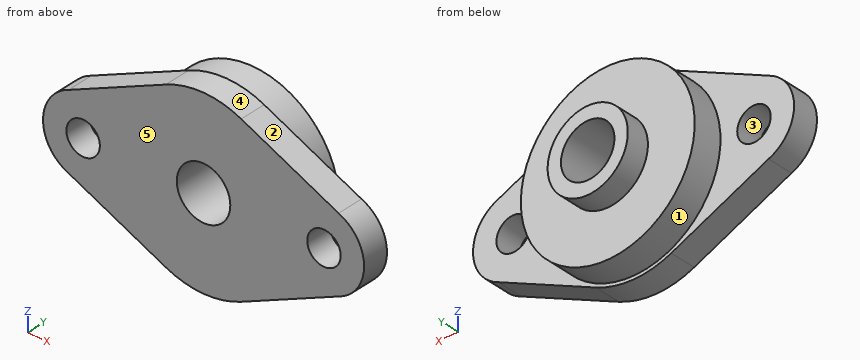
from build123d import *

# Parameters (mm, degrees)
SKETCH1_R           = 2.5
SKETCH1_R_2         = 4
BOSS_EXTRUDE1_DEPTH = 4
SKETCH2_R           = 13
SKETCH2_R_2         = 4
BOSS_EXTRUDE2_DEPTH = 4.5
SKETCH3_R           = 6
SKETCH3_R_2         = 4
BOSS_EXTRUDE3_DEPTH = 3.5


with BuildPart() as part:
    # Sketch1 → Boss-Extrude1 (new body)
    with BuildSketch(Plane(origin=(0, 0, 0), x_dir=(1, 0, 0), z_dir=(0, 1, 0))):
        with BuildLine():
            Line((-20.189639751, 5.586186334), (-5.632256707, 12.268972426))
            ThreePointArc((-5.632256707, 12.268972426), (0, 13.5), (5.632256707, 12.268972426))
            Line((5.632256707, 12.268972426), (20.189639751, 5.586186334))
            ThreePointArc((20.189639751, 5.586186334), (24, 0), (20.189639751, -5.586186334))
            Line((20.189639751, -5.586186334), (5.632256707, -12.268972426))
            ThreePointArc((5.632256707, -12.268972426), (0, -13.5), (-5.632256707, -12.268972426))
            Line((-5.632256707, -12.268972426), (-20.189639751, -5.586186334))
            ThreePointArc((-20.189639751, -5.586186334), (-24, 0), (-20.189639751, 5.586186334))
        make_face()
        with Locations((18, 0)):
            Circle(SKETCH1_R, mode=Mode.SUBTRACT)
        with Locations((-18, 0)):
            Circle(SKETCH1_R, mode=Mode.SUBTRACT)
        Circle(SKETCH1_R_2, mode=Mode.SUBTRACT)
    extrude(amount=BOSS_EXTRUDE1_DEPTH)

    # Sketch2 → Boss-Extrude2 (add)
    with BuildSketch(Plane(origin=(0, 4, 0), x_dir=(1, 0, 0), z_dir=(0, 1, 0))):
        Circle(SKETCH2_R)
        Circle(SKETCH2_R_2, mode=Mode.SUBTRACT)
    extrude(amount=BOSS_EXTRUDE2_DEPTH)

    # Sketch3 → Boss-Extrude3 (add)
    with BuildSketch(Plane(origin=(0, 8.5, 0), x_dir=(1, 0, 0), z_dir=(0, 1, 0))):
        Circle(SKETCH3_R)
        Circle(SKETCH3_R_2, mode=Mode.SUBTRACT)
    extrude(amount=BOSS_EXTRUDE3_DEPTH)


solid = part.part
For this review, take the finished solid that the model builds, in its own axes (mm). Face numbers are marked on the shaded views. A direction names the side the tool comes from. Give positions to 0.01 mm unless a question says otherwise; leave off trailing zeros. Order: outer loops, then holes, each group sorted by start corner. A loop starts at its lowest first (then second) coordinate and runs counter-clockwise, first axis right, second up. Notation, with made-up numbers: (-16, 60.25) - (9, 60.25) arc R9 cw to (9, 74.25) - close; hole circle Ø8 at (-28.5, -25.75). An arc over 180 degrees is marked (long way). Answer as a JSON object with one key per item and string values. Group by question number.
Item 1: Take a section at D-D on x = -5. Give the boundary of the cut face in (y, z).
Item 2: Take a section at B-B on z = 0. Give the boundary of the cut face in (x, y), and give its area (3 significant figures).
Item 3: Wall thickness on line 1 along Z through (x, y) = (0, 6.25); line 2 along Z through (x, y) = (0, 9); line 3 along Y through (x, z) = (11.5, -0.25): over which ranges is each line inside the solid? List them lowest first.
Item 4: Draft analysis for pull direction Z (two halves, no side actions). For the marked faces 3, 4 and 5, state which applies: pulls with the +Z half, pulls with the -Z half, needs draft (parallel to the pull), parting line crosses it, or undercut.
Item 5: Clearance check with flat-ended pins moving along their axes: pin 1 Ø3 at (x, z) = (-6.5, -8) entering from +Y; pin 2 Ø7 at (x, z) = (0, 0) entering from +Y; pin 3 Ø4 at (y, z) = (3.5, 3) entering from +X. State where each tip first meets the part, or that it passes through.
Item 6: Take a section at A-A on x = 0. Give the boundary of the cut face in (y, z).
Item 7: Machinability: for the marked faces 1 and 2, which of the approach directions +Z, -Z, +X, -X, +Y, -Y give a long, thin tool a straight path to every point of the face, cutting with its end or side? Answer none if there is none.
Item 8: Take a section at C-C on z = -11.25. Give the boundary of the cut face in (x, y).
Reported:
{
 "1": {"outline": "(0, -12.54) - (4, -12.54) - (4, -12) - (8.5, -12) - (8.5, -3.32) - (12, -3.32) - (12, 3.32) - (8.5, 3.32) - (8.5, 12) - (4, 12) - (4, 12.54) - (0, 12.54) - close"},
 "2": {"outline": "(-24, 0) - (-20.5, 0) - (-20.5, 4) - (-24, 4) - close; (-15.5, 0) - (-4, 0) - (-4, 12) - (-6, 12) - (-6, 8.5) - (-13, 8.5) - (-13, 4) - (-15.5, 4) - close; (4, 0) - (15.5, 0) - (15.5, 4) - (13, 4) - (13, 8.5) - (6, 8.5) - (6, 12) - (4, 12) - close; (20.5, 0) - (24, 0) - (24, 4) - (20.5, 4) - close", "area": "215 mm^2"},
 "3": {"line 1": "-13 to -4, 4 to 13", "line 2": "-6 to -4, 4 to 6", "line 3": "0 to 8.5"},
 "4": {"face 3": "undercut", "face 4": "pulls with the +Z half", "face 5": "needs draft"},
 "5": {"pin 1": "y = 8.5", "pin 2": "through", "pin 3": "x = 23.92"},
 "6": {"outline": "(0, -13.5) - (4, -13.5) - (4, -13) - (8.5, -13) - (8.5, -6) - (12, -6) - (12, -4) - (0, -4) - close; (0, 4) - (12, 4) - (12, 6) - (8.5, 6) - (8.5, 13) - (4, 13) - (4, 13.5) - (0, 13.5) - close"},
 "7": {"face 1": "+Y", "face 2": "+Z, +X, +Y, -Y"},
 "8": {"outline": "(-7.85, 0) - (7.85, 0) - (7.85, 4) - (6.51, 4) - (6.51, 8.5) - (-6.51, 8.5) - (-6.51, 4) - (-7.85, 4) - close"}
}
